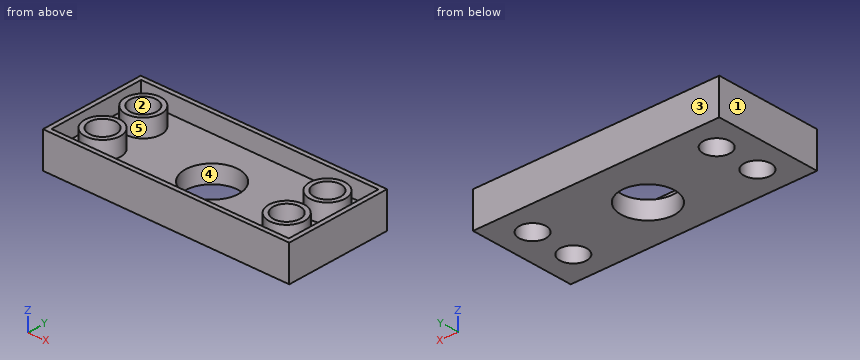
```python
from build123d import *

# Parameters (mm, degrees)
SKETCH1_W           = 169.85
SKETCH1_H           = 69.85
SKETCH1_R           = 9.525
SKETCH1_R_2         = 19.05
BOSS_EXTRUDE1_DEPTH = 12.7
SKETCH2_R           = 12.7
SKETCH2_R_2         = 9.525
BOSS_EXTRUDE2_DEPTH = 12.7
SKETCH3_W           = 176.2
SKETCH3_H           = 76.2
SKETCH3_W_2         = 169.85
SKETCH3_H_2         = 69.85
BOSS_EXTRUDE3_DEPTH = 25.4


with BuildPart() as part:
    # Sketch1 → Boss-Extrude1 (new body)
    with BuildSketch(Plane.XY):
        with Locations((46.032710784, 129.625650191)):
            Rectangle(SKETCH1_W, SKETCH1_H)
        with Locations((-19.842289216, 145.500650191)):
            Circle(SKETCH1_R, mode=Mode.SUBTRACT)
        with Locations((-19.842289216, 113.750650191)):
            Circle(SKETCH1_R, mode=Mode.SUBTRACT)
        with Locations((111.907710784, 145.500650191)):
            Circle(SKETCH1_R, mode=Mode.SUBTRACT)
        with Locations((111.907710784, 113.750650191)):
            Circle(SKETCH1_R, mode=Mode.SUBTRACT)
        with Locations((46.032710784, 127.370341001)):
            Circle(SKETCH1_R_2, mode=Mode.SUBTRACT)
    extrude(amount=BOSS_EXTRUDE1_DEPTH)

    # Sketch2 → Boss-Extrude2 (add)
    with BuildSketch(Plane.XY.offset(12.7)):
        with Locations((111.907710784, 145.500650191)):
            Circle(SKETCH2_R)
        with Locations((111.907710784, 145.500650191)):
            Circle(SKETCH2_R_2, mode=Mode.SUBTRACT)
        with Locations((111.907710784, 113.750650191)):
            Circle(SKETCH2_R)
        with Locations((111.907710784, 113.750650191)):
            Circle(SKETCH2_R_2, mode=Mode.SUBTRACT)
        with Locations((-19.842289216, 113.750650191)):
            Circle(SKETCH2_R)
        with Locations((-19.842289216, 113.750650191)):
            Circle(SKETCH2_R_2, mode=Mode.SUBTRACT)
        with Locations((-19.842289216, 145.500650191)):
            Circle(SKETCH2_R)
        with Locations((-19.842289216, 145.500650191)):
            Circle(SKETCH2_R_2, mode=Mode.SUBTRACT)
    extrude(amount=BOSS_EXTRUDE2_DEPTH)

    # Sketch3 → Boss-Extrude3 (add)
    with BuildSketch(Plane(origin=(0, 0, 0), x_dir=(-1, 0, 0), z_dir=(0, 0, -1))):
        with Locations((-46.032710784, 129.625650191)):
            Rectangle(SKETCH3_W, SKETCH3_H)
        with Locations((-46.032710784, 129.625650191)):
            Rectangle(SKETCH3_W_2, SKETCH3_H_2, mode=Mode.SUBTRACT)
    extrude(amount=-BOSS_EXTRUDE3_DEPTH)


solid = part.part
```
Source: CAD feature listing. Evaluate the final solid. Frame: model axes, mm. Face numbers are marked on the shaded views. A direction names the side the tool comes from. Coordinates: 2 decimals unless noted, no trailing zeros. Write each loop counter-clockwise with the first axis right and the second up, starting at its lowest first coordinate (ties: lowest second). Pieces come first, ordered by that corner, then holes. Notation, with made-up numbers: (20, 15.25) -> (25, 15.25) arc R16 ccw to (25, 31.25) -> close; hole circle Ø4 at (79.5, 39). An arc over 180 degrees is marked (long way). Return JSON: item names as keys, results as strings. Group by question number.
1) Section query D-D, the plane x = 8.5. Return loops of the section in (y, z), plus the area to 3 significant figures.
2) Section query B-B, the plane z = 21. State how many separate pieces and enclosed holes the cut face has, plus the area to 3 significant figures.
3) Section query C-C, the plane x = 32. Return loops of the section in (y, z).
4) Set-up query: the marked faces 4 and 5. Return all of +Z, -Z, +X, -X, +Y, -Y with unobstructed straight access to the full face (end or side cutting, diameter ignored); none if empty.
5) Mould query, pull axis Y, two halves, no side actions, for the marked faces 1, 2 and 3. Classes: +Y half, -Y half, draft (parallel to the pull), parting line (faces both ways), or undercut.
6) Section query A-A, the plane x = 104. Return loops of the section in (y, z), plus the area to 3 significant figures.
7) Ray query, line 1 along Y through (x, z) = (-28, 12); line 2 along X through (y, z) = (96, 21.5); line 3 along X through (y, z) = (147, 17.75). Return the intervals inside material, ascending.
From the geometry:
{
 "1": {"outline": "(91.53, 0) -> (167.73, 0) -> (167.73, 25.4) -> (164.55, 25.4) -> (164.55, 12.7) -> (94.7, 12.7) -> (94.7, 25.4) -> (91.53, 25.4) -> close", "area": "1,050 mm²"},
 "2": {"separate pieces": "5", "enclosed holes": "5", "area": "2,450 mm²"},
 "3": {"outline": "(91.53, 0) -> (114.49, 0) -> (114.49, 12.7) -> (94.7, 12.7) -> (94.7, 25.4) -> (91.53, 25.4) -> close; (140.25, 0) -> (167.73, 0) -> (167.73, 25.4) -> (164.55, 25.4) -> (164.55, 12.7) -> (140.25, 12.7) -> close"},
 "4": {"face 4": "+Z, -Z", "face 5": "+Z"},
 "5": {"face 1": "draft", "face 2": "undercut", "face 3": "+Y half"},
 "6": {"outline": "(91.53, 0) -> (108.44, 0) -> (108.44, 25.4) -> (103.81, 25.4) -> (103.81, 12.7) -> (94.7, 12.7) -> (94.7, 25.4) -> (91.53, 25.4) -> close; (119.06, 0) -> (140.19, 0) -> (140.19, 25.4) -> (135.56, 25.4) -> (135.56, 12.7) -> (123.69, 12.7) -> (123.69, 25.4) -> (119.06, 25.4) -> close; (150.81, 0) -> (167.73, 0) -> (167.73, 25.4) -> (164.55, 25.4) -> (164.55, 12.7) -> (155.44, 12.7) -> (155.44, 25.4) -> (150.81, 25.4) -> close", "area": "1,010 mm²"},
 "7": {"line 1": "91.53 to 108.83, 118.67 to 140.58, 150.42 to 167.73", "line 2": "-42.07 to -38.89, 130.96 to 134.13", "line 3": "-42.07 to -38.89, -32.45 to -29.25, -10.44 to -7.23, 99.3 to 102.5, 121.31 to 124.52, 130.96 to 134.13"}
}
